```python
from build123d import *

# Parameters (mm, degrees)
BOSS_EXTRUDE1_DEPTH = 43
CUT_EXTRUDE2_DEPTH  = 101.611036298
FILLET1_R           = 2.5


with BuildPart() as part:
    # Sketch1 → Boss-Extrude1 (new, symmetric)
    with BuildSketch(Plane.XY):
        Polygon((-46.5, 39.0875), (-46.5, 29.0875), (-19.625, 29.0875), (-19.625, -29.0875), (-46.5, -29.0875), (-46.5, -39.0875), (0, -39.0875), (0, 39.0875), align=None)
    extrude(amount=BOSS_EXTRUDE1_DEPTH, both=True)

    # Sketch2 → Cut-Extrude2 (cut, through all)
    with BuildSketch(Plane(origin=(0, 39.0875, 0), x_dir=(1, 0, 0), z_dir=(0, 1, 0))):
        with BuildLine():
            Line((-36.625, -43), (-36.625, 19))
            ThreePointArc((-36.625, 19), (-33.125, 22.5), (-29.625, 19))
            Line((-29.625, 19), (-29.625, -43))
            Line((-29.625, -43), (-36.625, -43))
        make_face()
    extrude(amount=-CUT_EXTRUDE2_DEPTH, mode=Mode.SUBTRACT)

    # Fillet1
    fillet1_edges = [part.edges().sort_by_distance(p)[0] for p in [
        (-46.5, 34.0875, -43),
        (-46.5, -34.0875, 43),
        (0, 0, 43),
        (0, 0, -43),
        (-46.5, 34.0875, 43),
        (-46.5, -34.0875, -43),
    ]]
    fillet(fillet1_edges, radius=FILLET1_R)


solid = part.part
```
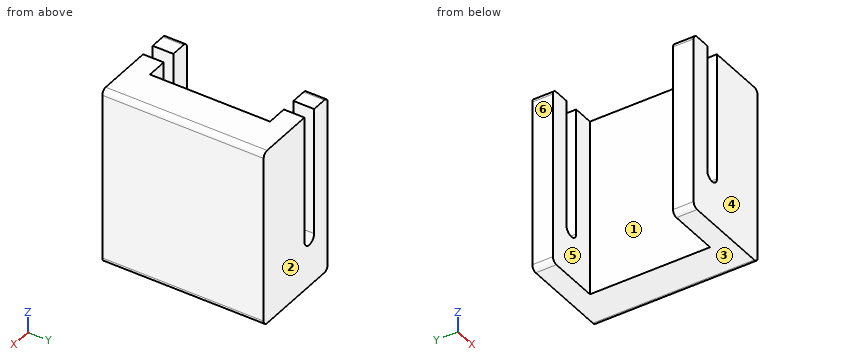
Read the model definition and answer for the solid it produces. Units are mm, in the model's axes. Face numbers are marked on the shaded views. A direction names the side the tool comes from. Coordinates: 2 decimals unless noted, no trailing zeros. Loops run counter-clockwise (first coordinate to the right, second up) from the corner with the lowest first, then second, coordinate; pieces in that order, holes last. Notation, with made-up numbers: (-20.5, -30.75) -> (30.5, -30.75) arc R35 ccw to (30.5, 4.25) -> close; hole circle Ø3 at (-18.75, 26.25). An arc over 180 degrees is marked (long way). Return JSON: item names as keys, results as strings.
Item 1: Find section B-B (x = -21). Determine the outline of the cut face in (y, z).
Answers:
{"outline": "(-39.09, -43) -> (-29.09, -43) -> (-29.09, 43) -> (-39.09, 43) -> close; (29.09, -43) -> (39.09, -43) -> (39.09, 43) -> (29.09, 43) -> close"}
Item 2: Find section C-C (y = 3). Determine the outline of the cut face in (x, z) (3 decimals).
Answers:
{"outline": "(-19.625, -43) -> (-2.5, -43) arc R2.5 ccw to (0, -40.5) -> (0, 40.5) arc R2.5 ccw to (-2.5, 43) -> (-19.625, 43) -> close"}
Item 3: For a pull along Y with two mould halves and no side action, classify the marked faces 1, 2, 3 and 4 as +Y half, -Y half, draft (parallel to the pull), parting line (faces both ways), or undercut.
Answers:
{"face 1": "undercut", "face 2": "+Y half", "face 3": "draft", "face 4": "-Y half"}
Item 4: A flat-ended cylindrical pin translates along its axis: P1, Ø1, axis at y = -4.5, z = 1, coming from the -X side (3 decimals). Find the tip coordinate at first contact, or state that the pin passes through.
Answers:
{"P1": "stops at x = -19.625"}
Item 5: Find the intervals of material crossed by probe 1 along X at (y, z) = (31.5, 14.5) (3 decimals); probe 2 along Y at (x, z) = (-25, 4.5); probe 3 along X at (y, z) = (14.5, -24.5) (3 decimals), in increasing order.
Answers:
{"probe 1": "x = -46.5 to -36.625, -29.625 to 0", "probe 2": "y = -39.09 to -29.09, 29.09 to 39.09", "probe 3": "x = -19.625 to 0"}
Item 6: Find section A-A (z = 0.5). Determine the outline of the cut face in (x, y) (1 decimal), plus the area to 3 significant figures.
Answers:
{"outline": "(-46.5, -39.1) -> (-36.6, -39.1) -> (-36.6, -29.1) -> (-46.5, -29.1) -> close; (-46.5, 29.1) -> (-36.6, 29.1) -> (-36.6, 39.1) -> (-46.5, 39.1) -> close; (-29.6, -39.1) -> (0, -39.1) -> (0, 39.1) -> (-29.6, 39.1) -> (-29.6, 29.1) -> (-19.6, 29.1) -> (-19.6, -29.1) -> (-29.6, -29.1) -> close", "area": "1,930 mm2"}
Item 7: For the marked faces 5 and 6, determine the directions among +Z, -Z, +X, -X, +Y, -Y from which every point of the face is accessible in a straight line to the end or side of a thin tool.
Answers:
{"face 5": "+Z, -Z, -X", "face 6": "+Z, -Z, -X, +Y, -Y"}
